Design review of the part shown in the three views and the two pictorial views. Dimensions are in mm from the part's minimum x, y and z. Coordinates: 2 decimals unless noted, no trailing zeros. Loops run counter-clockwise (first coordinate to the right, second up) from the corner with the lowest first, then second, coordinate; pieces in that order, holes last. Notation, with made-up numbers: (22, -39) -> (42, -39) arc R8 cw to (42, -27) -> close; hole circle Ø9 at (55.5, 17). An arc over 180 degrees is marked (long way). Answer in a Markdown table with one row per item.
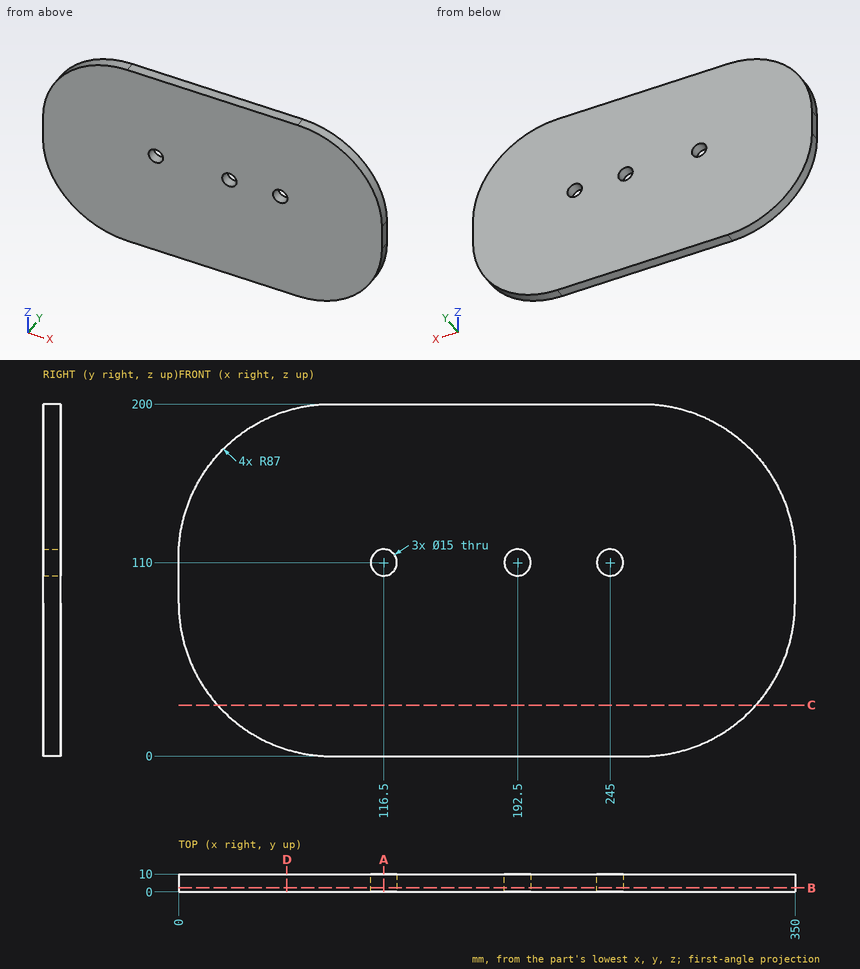
Item 1: Take a section at A-A, the plane x = 116.5. State the section outline as (y, z) points, and give its area (3 significant figures).
Worked answers:
| item | result |
|---|---|
| outline | (0, 0) -> (10, 0) -> (10, 102.5) -> (0, 102.5) -> close; (0, 117.5) -> (10, 117.5) -> (10, 200) -> (0, 200) -> close |
| area | 1,850 mm² |
Item 2: For L1, parallel to X at y = 8.5, z = 109; L2, parallel to Z at x = 245, y = 8.25; L3, parallel to X at y = 7.25, z = 84, list the stretches that pass through material, from the lowest coordinate up.
Worked answers:
| item | result |
|---|---|
| L1 | 0 to 109.07, 123.93 to 185.07, 199.93 to 237.57, 252.43 to 350 |
| L2 | 0 to 102.5, 117.5 to 200 |
| L3 | 0.05 to 349.95 |
Item 3: Take a section at B-B, the plane y = 2.25. State the section outline as (x, z) points.
Worked answers:
| item | result |
|---|---|
| outline | (0, 87) arc R87 ccw to (87, 0) -> (263, 0) arc R87 ccw to (350, 87) -> (350, 113) arc R87 ccw to (263, 200) -> (87, 200) arc R87 ccw to (0, 113) -> close; hole circle Ø15 at (116.5, 110); hole circle Ø15 at (192.5, 110); hole circle Ø15 at (245, 110) |
Item 4: Take a section at C-C, the plane z = 29. State the section outline as (x, y) points, and give its area (3 significant figures).
Worked answers:
| item | result |
|---|---|
| outline | (22.15, 0) -> (327.85, 0) -> (327.85, 10) -> (22.15, 10) -> close |
| area | 3,060 mm² |
Item 5: Take a section at D-D, the plane x = 61.5. State the section outline as (y, z) points, and give its area (3 significant figures).
Worked answers:
| item | result |
|---|---|
| outline | (0, 3.82) -> (10, 3.82) -> (10, 196.18) -> (0, 196.18) -> close |
| area | 1,920 mm² |
Item 6: Insertion check: pin 1 (1 mm diameter, centred on y = 2.5, z = 25, fed in from -X); pin 2 (3 mm diameter, centred on x = 59, y = 2.5, fed in from +Z); pin 3 (3 mm diameter, centred on x = 49, z = 70.5, fed in from -Y); pin 4 (1.5 mm diameter, centred on y = 6, z = 115.5, fed in from +X). Each pin has a flat end and moves straight along its axis. Give the tip position at first contact, or say it passes through.
Worked answers:
| item | result |
|---|---|
| pin 1 | x = 25.46 |
| pin 2 | z = 195.87 |
| pin 3 | y = 0 |
| pin 4 | x = 349.98 |
